Check sheet for the modelled part. Datum: model origin and axes. Units: mm. A direction names the side the tool comes from. Round coordinates to 2 decimals unless told otherwise and drop trailing zeros. Order: outer loops, then holes, each group sorted by start corner. A loop starts at its lowest first (then second) coordinate and runs counter-clockwise, first axis right, second up.
Autodesk Inventor part; units mm, degrees
ref_plane "YZ Plane" through (0, 0, 0) normal (1, 0, 0) x (0, 1, 0)
ref_plane "XZ Plane" through (0, 0, 0) normal (0, 1, 0) x (-1, 0, 0)
ref_plane "XY Plane" through (0, 0, 0) normal (0, 0, 1) x (1, 0, 0)
sketch "Sketch1" plane through (0, 0, 0) normal (0, 1, 0) x (-1, 0, 0)
  line L0 (0, 0) -> (0, -30)
  line L1 (0, -30) -> (-30, -30)
  line L2 (-30, -30) -> (-30, 0)
  line L3 (-30, 0) -> (0, 0)
  dimension "d0" = 30
  dimension "d1" = 30
extrude "Extrusion1" add sketch "Sketch1" along normal blind 2
sketch "Sketch2" plane through (0, 2, 0) normal (0, 1, 0) x (1, 0, 0)
  line L0 (0, 30) -> (0, 0)
  line L1 (25.05, 0) -> (30, 0)
  line L2 (30, 0) -> (30, 30)
  line L3 (30, 0) -> (30, 30)
  line L4 (30, 30) -> (25.05, 30)
  line L5 (25.05, 30) -> (25.05, 0)
  line L6 (30, 0) -> (30, 30)
  line L7 (0, 0) -> (30, 0)
  line L8 (30, 30) -> (0, 30)
  line L9 (4.95, 0) -> (0, 0)
  line L10 (0, 0) -> (0, 30)
  line L11 (0, 30) -> (4.95, 30)
  line L12 (4.95, 30) -> (4.95, 0)
  point P0 (4.95, 0)
extrude "Extrusion2" add sketch "Sketch2" along normal blind 1.56 contours L8 L12 L7 L0 | L4 L2 L1 L5
sketch "Sketch3" plane through (0, 3.56, 0) normal (0, 1, 0) x (1, 0, 0)
  line L0 (0, 30) -> (0, 0)
  line L1 (0, 0) -> (0, 30)
  line L2 (0, 30) -> (5.95, 30)
  line L3 (5.95, 30) -> (5.95, 0)
  line L4 (5.95, 0) -> (0, 0)
  line L5 (4.95, 0) -> (25.05, 0)
  line L6 (25.05, 30) -> (4.95, 30)
  line L7 (30, 30) -> (30, 0)
  line L8 (30, 0) -> (30, 30)
  line L9 (30, 30) -> (24.05, 30)
  line L10 (24.05, 30) -> (24.05, 0)
  line L11 (24.05, 0) -> (30, 0)
  point P0 (24.05, 0)
  dimension "d8" = 30
  dimension "d9" = 5.95
extrude "Extrusion3" add sketch "Sketch3" along normal blind 1 contours L2 L3 L4 L0 | L6 L9 L7 L11 L5 L10
sketch "Sketch5" plane through (0, 4.56, 0) normal (0, 1, 0) x (1, 0, 0)
  circle A0 centre (2.975, 2.5) radius 1.55
  circle A1 centre (27.025, 27.5) radius 1.55
  line L0 (30, 30) -> (24.05, 30)
  line L1 (30, 0) -> (30, 30)
  line L2 (0, 30) -> (0, 0)
  line L3 (0, 0) -> (5.95, 0)
  dimension "d13" = 3.1
  dimension "d14" = 3.1
  dimension "d15" = 2.5
  dimension "d16" = 2.975
  dimension "d18" = 2.975
  dimension "d19" = 2.5
extrude "Extrusion4" cut sketch "Sketch5" against normal blind 10
sketch "Sketch6" plane through (0, 2, 0) normal (0, 1, 0) x (1, 0, 0)
  circle A0 centre (27.025, 27.5) radius 1.55
  point P0 (0, 0)
properties part number "rplidar_adapter_board_holder" material "PET Plastic"
1) Gauge pin test, flat end, axial feed: pin 1 (6 mm diameter, centred on x = 16.5, z = -11.5, fed in from +Y). Record the tip position at first contact, or that the pin passes through.
2) Scan lines: line 1 (X direction, y = 3.2, z = -2.5) (3 decimals); line 2 (X direction, y = 2.3, z = -27.5) (3 decimals); line 3 (X direction, y = 2.2, z = -25.25). Record each from-to range of solid material in increasing order.
3) Sectioned sample at A-A on y = 2.75. Record the cut outline in (x, z) (3 decimals), and give its area (3 significant figures).
4) Sectioned sample at B-B on z = -2.5. Record the cut outline in (x, y) (3 decimals), and give its area (3 significant figures).
5) Sectioned sample at C-C on z = -16. Record the cut outline in (x, y), and give its area (3 significant figures).
6) Draft check along Y on faces 1 (the face through (15, 0, -15)), 2 (the face through (15.2, 1.7, 0)), 3 (the face through (5.4, 3.56, -15.2)). Enter one of: pulls with the +Y half, pulls with the -Y half, needs draft (parallel to the pull), parting line crosses it, or undercut.
7) Sectioned sample at D-D on x = 10.75. Record the cut outline in (y, z).
8) Set-up check for faces 4 (the face through (4.95, 3, -15)), 5 (the face through (3, 4.56, -15)), 6 (the face through (24.05, 4, -15)): record each of +Z, -Z, +X, -X, +Y, -Y from which the full face is reachable in a straight line by a thin tool's end or side.
Values found:
1. pin 1: stops at y = 2
2. line 1: x = 0 to 1.425, 4.525 to 4.95, 25.05 to 30
2. line 2: x = 0 to 4.95, 25.05 to 25.475, 28.575 to 30
2. line 3: x = 0 to 4.95, 25.05 to 30
3. outline: (0, -30) - (4.95, -30) - (4.95, 0) - (0, 0) - close; (25.05, -30) - (30, -30) - (30, 0) - (25.05, 0) - close; hole circle Ø3.1 at (2.975, -2.5); hole circle Ø3.1 at (27.025, -27.5)
3. area: 282 mm2
4. outline: (0, 0) - (1.425, 0) - (1.425, 4.56) - (0, 4.56) - close; (4.525, 0) - (30, 0) - (30, 4.56) - (24.05, 4.56) - (24.05, 3.56) - (25.05, 3.56) - (25.05, 2) - (4.95, 2) - (4.95, 3.56) - (5.95, 3.56) - (5.95, 4.56) - (4.525, 4.56) - close
4. area: 73.2 mm2
5. outline: (0, 0) - (30, 0) - (30, 4.56) - (24.05, 4.56) - (24.05, 3.56) - (25.05, 3.56) - (25.05, 2) - (4.95, 2) - (4.95, 3.56) - (5.95, 3.56) - (5.95, 4.56) - (0, 4.56) - close
5. area: 87.3 mm2
6. face 1: pulls with the -Y half
6. face 2: needs draft
6. face 3: undercut
7. outline: (0, -30) - (2, -30) - (2, 0) - (0, 0) - close
8. face 4: +Z, -Z
8. face 5: +Z, -Z, +X, -X, +Y
8. face 6: +Z, -Z, +Y
